Autodesk Inventor part; units mm, degrees
ref_plane "YZ Plane" through (0, 0, 0) normal (1, 0, 0) x (0, 1, 0)
ref_plane "XZ Plane" through (0, 0, 0) normal (0, 1, 0) x (-1, 0, 0)
ref_plane "XY Plane" through (0, 0, 0) normal (0, 0, 1) x (1, 0, 0)
sketch "スケッチ1" plane through (0, 0, 0) normal (1, 0, 0) x (0, 1, 0)
  line L0 (0, 125) -> (0, -125)
  line L1 (-193.7075, 0) -> (764.5712, 0)
  arc A0 (0, 125) -> (0, -125) centre (627.6743, 0) ccw
  arc A1 (0, 125) -> (-45.1737, 25) centre (79.0119, 29.1041) ccw
  arc A2 (-45.1737, 25) -> (0, -125) centre (259.9333, 35.0832) ccw
  point P0 (0, 0)
  point P1 (0, 0)
  dimension "d0" = 250
  dimension "d1" = 640
  dimension "d16" = 100
extrude "押し出し4" add sketch "スケッチ1" along normal mid plane 50 contours A0 L1 A2 A1 | A0 A2 L1
fillet "フィレット3" radius 5 1 edges at (0, 0, 125)
fillet "フィレット3" radius 3 1 edges at (0, 0, -125)
sketch "スケッチ4" plane through (25, 0, 0) normal (1, 0, 0) x (0, 0, -1)
  circle A0 centre (23.3804, -26.1259) radius 6
  arc A1 (109.8042, -8.7665) -> (107.8747, -3.1688) centre (108.3804, -6.1259) ccw
  point P0 (0, 0)
  dimension "d21" = 12
  dimension "d22" = 85
  dimension "d23" = 20
extrude "押し出し5" cut sketch "スケッチ4" against normal through all
properties part number "styro_50_sub" material "ポリスチレン"
Can you work these out from the model? Positions are in its coordinate system, mm. Round coordinates to 2 decimals unless told otherwise and drop trailing zeros. Write each loop counter-clockwise with the first axis right and the second up, starting at its lowest first coordinate (ties: lowest second). Pieces come first, ordered by that corner, then holes. Notation, with made-up numbers: (28.5, 53) -> (58.5, 53) arc R8 cw to (58.5, 63) -> close; hole circle Ø3 at (4.5, 55). An arc over 180 degrees is marked (long way). Use one line per item in the form item = value. Start each with the question number.
Q1. I'm going to push flat-ended pins straight in: P1, Ø6, axis at x = 6, z = 66, coming from the -Y side; P2, Ø4, axis at x = 7.5, z = -80, coming from the -Y side; P3, Ø1.5, axis at x = -11, y = -34, coming from the +Z side. Where does each tip first touch, or does it pass through?
Q2. Imagine slicing it at B-B (z = -83). Please give me the cut outline in (x, y), then the cut area to 3 significant figures.
Q3. Imagine slicing it at A-A (y = -29). Please give me the cut outline in (x, z).
Q4. If I drill on probe 1 along Y at (x, z) = (-22.5, 91.5); probe 2 along Y at (x, z) = (-13.5, -7); probe 3 along Z at (x, y) = (-18, -13), over which ranges is the centre line in solid material (lowest first)? Write a range as [from, to].
Q5. Imagine slicing it at C-C (z = 47). Please give me the cut outline in (x, y).
Worked out:
q1.P1 = -40.53
q1.P2 = -23.62
q1.P3 = 82.36
q2.outline = (-25, -21.58) -> (25, -21.58) -> (25, -6.92) -> (-25, -6.92) -> close
q2.area = 733 mm^2
q3.outline = (-25, -63.45) -> (25, -63.45) -> (25, -28.65) -> (-25, -28.65) -> close; (-25, -18.11) -> (25, -18.11) -> (25, 90.52) -> (-25, 90.52) -> close
q4.probe_1 = [-28.44, -5.75]
q4.probe_2 = [-42.43, -12.29]
q4.probe_3 = [-101.66, 112.61]
q5.outline = (-25, -43.95) -> (25, -43.95) -> (25, -10.6) -> (-25, -10.6) -> close
